Design review of the part shown in the three views and the two pictorial views. Dimensions are in mm from the part's minimum x, y and z. A direction names the side the tool comes from. Coordinates: 2 decimals unless noted, no trailing zeros. Order: outer loops, then holes, each group sorted by start corner. A loop starts at its lowest first (then second) coordinate and runs counter-clockwise, first axis right, second up. Notation, with made-up numbers: M 52.5,63 L 77.5,63 A20 ccw 77.5,99 Z; hole C 68.5,88.25 d1. An arc over 180 degrees is marked long. Use CSV: the item, a comma, the result in double quotes.
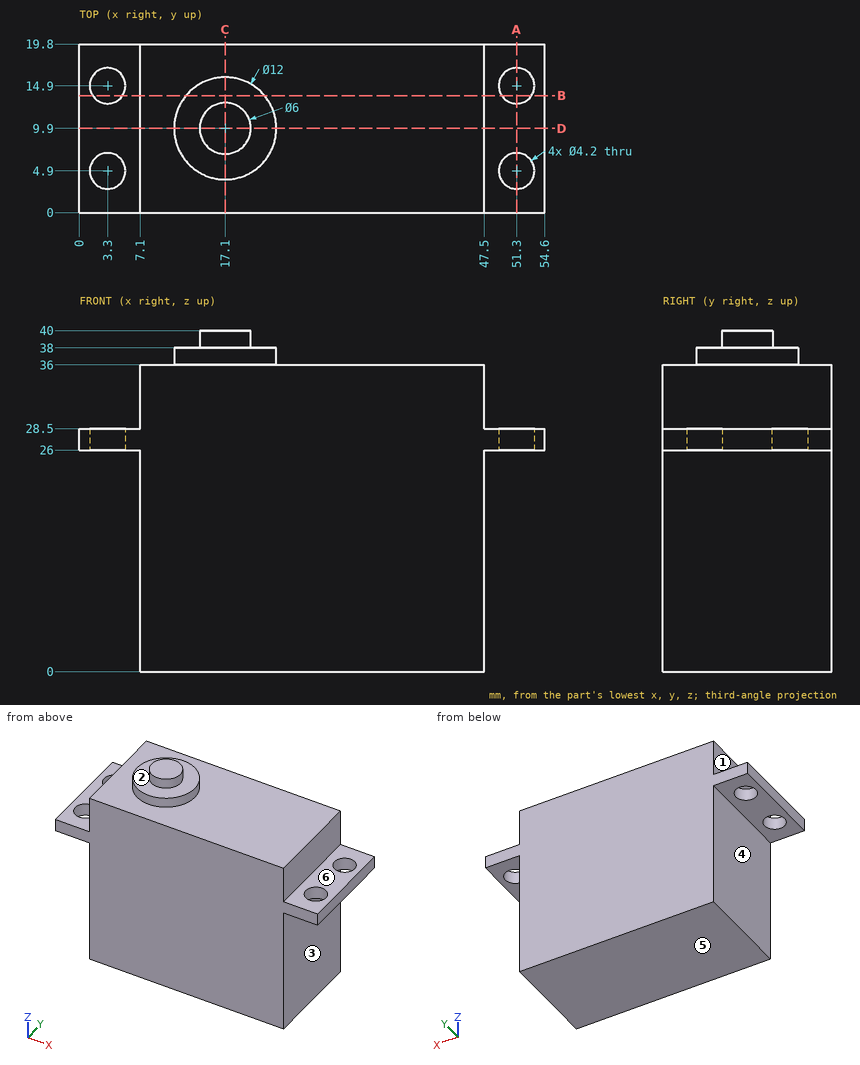
(1) Add section C-C on x = 17.1. State the section outline as (y, z) points.
The answers:
outline,"M 0,0 L 19.8,0 L 19.8,36 L 15.9,36 L 15.9,38 L 12.9,38 L 12.9,40 L 6.9,40 L 6.9,38 L 3.9,38 L 3.9,36 L 0,36 Z"
(2) Add section A-A on x = 51.3. State the section outline as (y, z) points.
The answers:
outline,"M 0,26 L 2.8,26 L 2.8,28.5 L 0,28.5 Z; M 7,26 L 12.8,26 L 12.8,28.5 L 7,28.5 Z; M 17,26 L 19.8,26 L 19.8,28.5 L 17,28.5 Z"
(3) Add section B-B on y = 13.75. State the section outline as (x, z) points, and give its area (3 significant figures).
The answers:
outline,"M 0,26 L 1.54,26 L 1.54,28.5 L 0,28.5 Z; M 5.06,26 L 7.1,26 L 7.1,0 L 47.5,0 L 47.5,26 L 49.54,26 L 49.54,28.5 L 47.5,28.5 L 47.5,36 L 21.7,36 L 21.7,38 L 12.5,38 L 12.5,36 L 7.1,36 L 7.1,28.5 L 5.06,28.5 Z; M 53.06,26 L 54.6,26 L 54.6,28.5 L 53.06,28.5 Z"
area,"1,490 mm2"
(4) Add section D-D on y = 9.9. State the section outline as (x, z) points, and give its area (3 significant figures).
The answers:
outline,"M 0,26 L 7.1,26 L 7.1,0 L 47.5,0 L 47.5,26 L 54.6,26 L 54.6,28.5 L 47.5,28.5 L 47.5,36 L 23.1,36 L 23.1,38 L 20.1,38 L 20.1,40 L 14.1,40 L 14.1,38 L 11.1,38 L 11.1,36 L 7.1,36 L 7.1,28.5 L 0,28.5 Z"
area,"1,530 mm2"
(5) Wall thickness on probe 1 along Y at (x, z) = (51.3, 27.3); probe 2 along Z at (x, y) = (48, 10.75); probe 3 along Z at (x, y) = (31, 11.25): over which ranges is each line inside the solid? List them lowest first.
The answers:
probe 1,"y = 0 to 2.8, 7 to 12.8, 17 to 19.8"
probe 2,"z = 26 to 28.5"
probe 3,"z = 0 to 36"
(6) Clearance check with flat-ended pins moving along their axes: P1, Ø8, axis at x = 49.5, y = 14, coming from the +Z side; P2, Ø3.5, axis at x = 2.5, y = 11.5, coming from the -Z side; P3, Ø1, axis at y = 13.5, z = 17, coming from the -X side. State where each tip first meets the part, or that it passes through.
The answers:
P1,"stops at z = 36"
P2,"stops at z = 26"
P3,"stops at x = 7.1"
(7) The part is to be moulded in two halves that separate along Z. For the marked faces 4, 5 and 6, say which applies: pulls with the +Z half, pulls with the -Z half, needs draft (parallel to the pull), parting line crosses it, or undercut.
The answers:
face 4,"needs draft"
face 5,"pulls with the -Z half"
face 6,"pulls with the +Z half"
(8) For the marked faces 1, 2 and 3, list the 3-axis set-ups (+Z, -Z, +X, -X, +Y, -Y) from which the entire face can be reached by the end or side of a thin tool; tool diameter is ignored.
The answers:
face 1,"+Z, -X, +Y, -Y"
face 2,"+Z"
face 3,"-Z, +X, +Y, -Y"
